The model under review builds one solid part; all positions refer to its coordinate system, in mm. A direction names the side the tool comes from. Give positions to 0.01 mm unless a question says otherwise; leave off trailing zeros. Order: outer loops, then holes, each group sorted by start corner. A loop starts at its lowest first (then second) coordinate and runs counter-clockwise, first axis right, second up.
```python
from build123d import *

# Parameters (mm, degrees)
SKETCH_1_R          = 2
EXTRUDE_1_DEPTH     = 1.5
SKETCH_2_R          = 1.6
CUT_EXTRUDE_1_DEPTH = 3


with BuildPart() as part:
    # 草图1 → 凸台-拉伸1 (new, symmetric)
    with BuildSketch(Plane.XY):
        with BuildLine():
            Line((-34.285, 24.845), (34.285, 24.845))
            ThreePointArc((34.285, 24.845), (37.488193719, 23.518193719), (38.815, 20.315))
            Line((38.815, 20.315), (38.815, -20.315))
            ThreePointArc((38.815, -20.315), (37.488193719, -23.518193719), (34.285, -24.845))
            Line((34.285, -24.845), (-34.285, -24.845))
            ThreePointArc((-34.285, -24.845), (-37.488193719, -23.518193719), (-38.815, -20.315))
            Line((-38.815, -20.315), (-38.815, 20.315))
            ThreePointArc((-38.815, 20.315), (-37.488193719, 23.518193719), (-34.285, 24.845))
        make_face()
        with Locations((34.29, 20.32)):
            Circle(SKETCH_1_R, mode=Mode.SUBTRACT)
        with Locations((34.29, -20.32)):
            Circle(SKETCH_1_R, mode=Mode.SUBTRACT)
        with Locations((-34.29, 20.32)):
            Circle(SKETCH_1_R, mode=Mode.SUBTRACT)
        with Locations((-34.285, -20.315)):
            Circle(SKETCH_1_R, mode=Mode.SUBTRACT)
    extrude(amount=EXTRUDE_1_DEPTH, both=True)

    # 草图2 → 切除-拉伸1 (cut)
    with BuildSketch(Plane.XY.offset(1.5)):
        with Locations((27.945, -19.005)):
            Circle(SKETCH_2_R)
        with Locations((24.135, -19.005)):
            Circle(SKETCH_2_R)
        with Locations((20.325, -19.005)):
            Circle(SKETCH_2_R)
        with BuildLine():
            Line((-31.255, 22.945), (16.005, 22.945))
            ThreePointArc((16.005, 22.945), (16.358553391, 22.798553391), (16.505, 22.445))
            Line((16.505, 22.445), (16.505, 15.235))
            ThreePointArc((16.505, 15.235), (16.358553391, 14.881446609), (16.005, 14.735))
            Line((16.005, 14.735), (-31.255, 14.735))
            ThreePointArc((-31.255, 14.735), (-31.608553391, 14.881446609), (-31.755, 15.235))
            Line((-31.755, 15.235), (-31.755, 22.445))
            ThreePointArc((-31.755, 22.445), (-31.608553391, 22.798553391), (-31.255, 22.945))
        make_face()
        with BuildLine():
            Line((-31.755, -22.445), (-31.755, -15.235))
            ThreePointArc((-31.755, -15.235), (-31.608553391, -14.881446609), (-31.255, -14.735))
            Line((-31.255, -14.735), (16.005, -14.735))
            ThreePointArc((16.005, -14.735), (16.358553391, -14.881446609), (16.505, -15.235))
            Line((16.505, -15.235), (16.505, -22.445))
            ThreePointArc((16.505, -22.445), (16.358553391, -22.798553391), (16.005, -22.945))
            Line((16.005, -22.945), (-31.255, -22.945))
            ThreePointArc((-31.255, -22.945), (-31.608553391, -22.798553391), (-31.755, -22.445))
        make_face()
        with BuildLine():
            Line((31.525, -7.685), (35.525, -7.685))
            ThreePointArc((35.525, -7.685), (35.701776695, -7.758223305), (35.775, -7.935))
            Line((35.775, -7.935), (35.775, -14.935))
            ThreePointArc((35.775, -14.935), (35.701776695, -15.111776695), (35.525, -15.185))
            Line((35.525, -15.185), (31.525, -15.185))
            ThreePointArc((31.525, -15.185), (31.348223305, -15.111776695), (31.275, -14.935))
            Line((31.275, -14.935), (31.275, -7.935))
            ThreePointArc((31.275, -7.935), (31.348223305, -7.758223305), (31.525, -7.685))
        make_face()
        with BuildLine():
            Line((7.485, 9.225), (19.685, 9.225))
            ThreePointArc((19.685, 9.225), (20.392106781, 8.932106781), (20.685, 8.225))
            Line((20.685, 8.225), (20.685, -8.225))
            ThreePointArc((20.685, -8.225), (20.392106781, -8.932106781), (19.685, -9.225))
            Line((19.685, -9.225), (7.485, -9.225))
            ThreePointArc((7.485, -9.225), (6.777893219, -8.932106781), (6.485, -8.225))
            Line((6.485, -8.225), (6.485, 8.225))
            ThreePointArc((6.485, 8.225), (6.777893219, 8.932106781), (7.485, 9.225))
        make_face()
    extrude(amount=-CUT_EXTRUDE_1_DEPTH, mode=Mode.SUBTRACT)


solid = part.part
```
Item 1: Draft analysis for pull direction Y (two halves, no side actions). For faces 1 (the cylindrical face through (37.453, 23.553, 0.021)), 2 (the cylindrical face through (-37.453, -23.553, 0.021)), 3 (the flat face through (13, 9.225, 0)), state which applies: released by +Y, released by -Y, zero draft, split by the parting line, or undercut.
Values found:
face 1: released by +Y
face 2: released by -Y
face 3: undercut
Item 2: Take a section at A-A (y = 6). Give the boundary of the cut face in (x, z) (3 decimals), and give its area (3 significant figures).
Values found:
outline: (-38.815, -1.5) - (6.485, -1.5) - (6.485, 1.5) - (-38.815, 1.5) - close; (20.685, -1.5) - (38.815, -1.5) - (38.815, 1.5) - (20.685, 1.5) - close
area: 190 mm2
Item 3: Take a section at C-C (y = 19.5). Give the boundary of the cut face in (x, z) (3 decimals), and give its area (3 significant figures).
Values found:
outline: (-38.815, -1.5) - (-36.114, -1.5) - (-36.114, 1.5) - (-38.815, 1.5) - close; (-32.466, -1.5) - (-31.755, -1.5) - (-31.755, 1.5) - (-32.466, 1.5) - close; (16.505, -1.5) - (32.466, -1.5) - (32.466, 1.5) - (16.505, 1.5) - close; (36.114, -1.5) - (38.815, -1.5) - (38.815, 1.5) - (36.114, 1.5) - close
area: 66.2 mm2
Item 4: Take a section at B-B (x = 4). Give the boundary of the cut face in (y, z) (3 decimals), and give its area (3 significant figures).
Values found:
outline: (-24.845, -1.5) - (-22.945, -1.5) - (-22.945, 1.5) - (-24.845, 1.5) - close; (-14.735, -1.5) - (14.735, -1.5) - (14.735, 1.5) - (-14.735, 1.5) - close; (22.945, -1.5) - (24.845, -1.5) - (24.845, 1.5) - (22.945, 1.5) - close
area: 99.8 mm2
Item 5: Take a section at D-D (z = -0.3). Give the number of separate pieces and of enclosed holes in the cut face, and give its area (3 significant figures).
Values found:
separate pieces: 1
enclosed holes: 11
area: 2,680 mm2
Item 6: For line 1 (Y direction, x = -14.5, z = 0.4) (3 decimals); line 2 (Y direction, x = 11, z = 1) (3 decimals); line 3 (Y direction, x = -34.29, z = 0.3) (3 decimals), list the stretches that pass through material, from the lowest coordinate up.
Values found:
line 1: y = -24.845 to -22.945, -14.735 to 14.735, 22.945 to 24.845
line 2: y = -24.845 to -22.945, -14.735 to -9.225, 9.225 to 14.735, 22.945 to 24.845
line 3: y = -24.845 to -22.315, -18.315 to 18.32, 22.32 to 24.845
Item 7: Clearance check with a flat-ended pin moving along its axis: pin 1 Ø4.5 at (x, y) = (34.29, -20.32) entering from -Z. State where the tip first meets the part, or that it passes through.
Values found:
pin 1: stops at z = -1.5
Item 8: For faces 4 (the flat face through (0, 24.845, 0)), 5 (the flat face through (-8, 22.945, 0)), list the 3-axis set-ups (+Z, -Z, +X, -X, +Y, -Y) from which the entire face can be reached by the end or side of a thin tool; tool diameter is ignored.
Values found:
face 4: +Z, -Z, +X, -X, +Y
face 5: +Z, -Z
